Read the model definition and answer for the solid it produces. Units are mm, in the model's axes. A direction names the side the tool comes from. Coordinates: 2 decimals unless noted, no trailing zeros. Order: outer loops, then holes, each group sorted by start corner. A loop starts at its lowest first (then second) coordinate and runs counter-clockwise, first axis right, second up. Notation, with made-up numbers: M -34.75,-38.75 L -3.75,-38.75 A6 cw -3.75,-29.75 Z; hole C -29.5,30 d5. An arc over 180 degrees is marked long. Write each question's results on one line, items separated by ' | '.
```python
from build123d import *

# Parameters (mm, degrees)
ESQUISSE1_R                = 100
BOSS_EXTRU_1_DEPTH         = 300
ESQUISSE2_R                = 30
ENL_V_MAT_EXTRU_1_DEPTH    = 300
CONG_3_R                   = 100
CONG_4_R                   = 10
ESQUISSE3_R                = 30
ENL_V_MAT_EXTRU_2_DEPTH    = 300
ESQUISSE4_R                = 10
ENL_V_MAT_EXTRU_3_DEPTH    = 100
R_P_TITION_LIN_AIRE1_COUNT = 3
R_P_TITION_LIN_AIRE1_PITCH = 120
CONG_5_R                   = 5


with BuildPart() as part:
    # Esquisse1 → Boss.-Extru.1 (new body)
    with BuildSketch(Plane.XY):
        with BuildLine():
            Line((0, 0), (900, 0))
            Line((900, 0), (900, 150))
            Line((900, 150), (730.278028845, 150))
            ThreePointArc((730.278028845, 150), (638.157551209, 188.157551209), (600, 280.278028845))
            Line((600, 280.278028845), (600, 375))
            Line((600, 375), (600, 527.089712385))
            Line((600, 527.089712385), (560, 527.089712385))
            Line((560, 527.089712385), (560, 600))
            Line((560, 600), (340, 600))
            Line((340, 600), (340, 527.089712385))
            Line((340, 527.089712385), (300, 527.089712385))
            Line((300, 527.089712385), (300, 375))
            Line((300, 375), (300, 291.936386231))
            ThreePointArc((300, 291.936386231), (256.792071963, 187.623220362), (152.478906094, 144.415292325))
            Line((152.478906094, 144.415292325), (0, 144.415292325))
            Line((0, 144.415292325), (0, 0))
        make_face()
        with Locations((450, 450)):
            Circle(ESQUISSE1_R, mode=Mode.SUBTRACT)
    extrude(amount=-BOSS_EXTRU_1_DEPTH)

    # Esquisse2 → Enlèv. mat.-Extru.1 (cut)
    with BuildSketch(Plane(origin=(0, 144.415292325, 0), x_dir=(1, 0, 0), z_dir=(0, 1, 0))):
        with Locations(Location((80, 250, 0), (0, 0, 270))):
            Circle(ESQUISSE2_R)
        with Locations(Location((80, 50, 0), (0, 0, 270))):
            Circle(ESQUISSE2_R)
    extrude(amount=-ENL_V_MAT_EXTRU_1_DEPTH, mode=Mode.SUBTRACT)

    # Congé3
    # the kernel refuses this fillet: 100 mm, written as the material it takes off along each edge
    with BuildSketch(Plane(origin=(340, 600, 240.652076177), x_dir=(1, 0, 0), z_dir=(0, 0, -1))) as cong_3_piece_1:
        with BuildLine():
            CenterArc((96.260830471, 100), CONG_3_R, 195.717657912, 74.282342088)
            Line((0, 72.910287615), (-1.925216609, 72.368493368))
            ThreePointArc((-1.925216609, 72.368493368), (-2, 36.455143808), (-2, 0))
            Line((-2, 0), (0, -2))
            Line((0, -2), (96.260830471, -2))
            Line((96.260830471, -2), (96.260830471, 0))
        make_face()
    extrude(amount=781.304152354, mode=Mode.SUBTRACT)
    with BuildSketch(Plane(origin=(560, 600, 240.652076177), x_dir=(0, -1, 0), z_dir=(0, 0, -1))) as cong_3_piece_2:
        with BuildLine():
            CenterArc((100, 96.260830471), CONG_3_R, 180, 74.282342088)
            Line((0, 96.260830471), (-2, 96.260830471))
            Line((-2, 96.260830471), (-2, 0))
            Line((-2, 0), (0, -2))
            ThreePointArc((0, -2), (36.455143808, -2), (72.368493368, -1.925216609))
            Line((72.368493368, -1.925216609), (72.910287615, 0))
        make_face()
    extrude(amount=781.304152354, mode=Mode.SUBTRACT)

    # Congé4
    cong_4_edges = [part.edges().sort_by_distance(p)[0] for p in [
        (300, 527.089712385, -150),
        (600, 527.089712385, -150),
    ]]
    fillet(cong_4_edges, radius=CONG_4_R)

    # Esquisse3 → Enlèv. mat.-Extru.2 (cut)
    with BuildSketch(Plane(origin=(0, 150, 0), x_dir=(1, 0, 0), z_dir=(0, 1, 0))):
        with Locations(Location((820, 250, 0), (0, 0, 270))):
            Circle(ESQUISSE3_R)
        with Locations(Location((820, 50, 0), (0, 0, 270))):
            Circle(ESQUISSE3_R)
    extrude(amount=-ENL_V_MAT_EXTRU_2_DEPTH, mode=Mode.SUBTRACT)

    # Esquisse4 → Enlèv. mat.-Extru.3 (cut)
    with BuildSketch(Plane(origin=(0, 527.089712385, 0), x_dir=(1, 0, 0), z_dir=(0, 1, 0))):
        with Locations(Location((573.784271885, 273.452208884, 0), (0, 0, 270))):
            Circle(ESQUISSE4_R)
        with Locations(Location((324.885406348, 273.452208884, 0), (0, 0, 270))):
            Circle(ESQUISSE4_R)
    enl_v_mat_extru_3 = extrude(amount=-ENL_V_MAT_EXTRU_3_DEPTH, mode=Mode.SUBTRACT)

    # Répétition linéaire1: Enlèv. mat.-Extru.3 ×3
    with Locations(*[(0, 0, i * R_P_TITION_LIN_AIRE1_PITCH) for i in range(1, R_P_TITION_LIN_AIRE1_COUNT)]):
        add(enl_v_mat_extru_3, mode=Mode.SUBTRACT)

    # Congé5
    cong_5_edges = [part.edges().sort_by_distance(p)[0] for p in [
        (900, 75, -300),
        (76.239453047, 144.415292325, 0),
        (256.792071963, 187.623220362, 0),
        (815.139014422, 150, -300),
        (325, 527.089712385, 0),
        (600, 398.683870615, 0),
        (638.157551209, 188.157551209, 0),
        (815.139014422, 150, 0),
        (638.157551209, 188.157551209, -300),
        (900, 75, 0),
        (0, 72.207646162, 0),
        (600, 398.683870615, -300),
        (0, 144.415292325, -150),
        (900, 150, -150),
        (325, 527.089712385, -300),
        (0, 72.207646162, -300),
        (256.792071963, 187.623220362, -300),
        (76.239453047, 144.415292325, -300),
        (300, 404.513049308, 0),
        (575, 527.089712385, 0),
        (597.071067812, 524.160780197, 0),
        (302.928932188, 524.160780197, 0),
        (300, 404.513049308, -300),
        (575, 527.089712385, -300),
        (597.071067812, 524.160780197, -300),
        (302.928932188, 524.160780197, -300),
    ]]
    fillet(cong_5_edges, radius=CONG_5_R)


solid = part.part
```
(1) Straight lines are drawn through the part: line 1 (X direction, y = 58, z = -50); line 2 (Y direction, x = 450, z = -199); line 3 (Y direction, x = 819, z = -18). For each, find the intervals that lie inside material, in ascending order.
Conclusion:
line 1: 0 to 50, 110 to 790, 850 to 900 | line 2: 0 to 350, 550 to 600 | line 3: 0 to 150
(2) For faces 5 (the flat face through (444, 171, -300)), 6 (the flat face through (80, 144.415, -148)), 7 (the cylindrical face through (316.014, 477.79, -268.838)), determine the directions among +Z, -Z, +X, -X, +Y, -Y from which every point of the face is accessible in a straight line to the end or side of a thin tool.
Conclusion:
face 5: -Z, +X, -X, +Y, -Y | face 6: +Z, -Z, -X, +Y | face 7: +Y
(3) The part is cut by section C-C, the plane x = 80. Write down the section's boundary in (y, z).
Conclusion:
outline: M 0,-300 L 139.42,-300 A5 ccw 144.42,-295 L 144.42,-280 L 0,-280 Z; M 0,-220 L 144.42,-220 L 144.42,-80 L 0,-80 Z; M 0,-20 L 144.42,-20 L 144.42,-5 A5 ccw 139.42,0 L 0,0 Z
(4) Given pin 1 (12 mm diameter, centred on x = 573.78, z = -273.45, fed in from +Y); pin 2 (2 mm diameter, centred on y = 193.5, z = -75, fed in from -X); pin 3 (5 mm diameter, centred on y = 475, z = -47.5, fed in from -X); pin 4 (6 mm diameter, centred on x = 543, y = 423, fed in from -Z), each flat-ended and moving along its own axis, determine where each tip first touches the part or whether it passes through.
Conclusion:
pin 1: y = 427.09 | pin 2: x = 261.45 | pin 3: x = 300 | pin 4: through
(5) The part is cut by section D-D, the plane y = 42.5. Write down the section's boundary in (x, z).
Conclusion:
outline: M 0,-295 A5 ccw 5,-300 L 895,-300 A5 ccw 900,-295 L 900,-5 A5 ccw 895,0 L 5,0 A5 ccw 0,-5 Z; hole C 80,-250 d60; hole C 80,-50 d60; hole C 820,-250 d60; hole C 820,-50 d60
(6) The part is cut by section B-B, the plane x = 450. Write down the section's boundary in (y, z), then the cut area to 3 significant figures.
Conclusion:
outline: M 0,-300 L 350,-300 L 350,0 L 0,0 Z; M 550,-300 L 600,-300 L 600,0 L 550,0 Z | area: 120,000 mm²
(7) The mould has two halves that part along Z. Classify faces 1 (the flat face through (444, 171, 0)), 2 (the cylindrical face through (315.123, 477.79, -35.62)), 3 (the flat face through (600, 397, -148)), 4 (the cylindrical face through (564.022, 477.79, -155.62)): pulls with the +Z half, pulls with the -Z half, needs draft (parallel to the pull), parting line crosses it, or undercut.
Conclusion:
face 1: pulls with the +Z half | face 2: undercut | face 3: needs draft | face 4: undercut
(8) The part is cut by section A-A, the plane z = -250. Write down the section's boundary in (x, y), then the cut area to 3 significant figures.
Conclusion:
outline: M 0,0 L 50,0 L 50,144.42 L 5,144.42 A5 ccw 0,139.42 Z; M 110,0 L 790,0 L 790,150 L 730.28,150 A130.28 cw 600,280.28 L 600,517.09 A10 ccw 590,527.09 L 560,527.09 A100 ccw 463.74,600 L 436.26,600 A100 ccw 340,527.09 L 310,527.09 A10 ccw 300,517.09 L 300,291.94 A147.52 cw 152.48,144.42 L 110,144.42 Z; M 850,0 L 900,0 L 900,145 A5 ccw 895,150 L 850,150 Z; hole C 450,450 d200 | area: 218,000 mm²
